from build123d import *

# Parameters (mm, degrees)
ESQUISSE2_R             = 3
ENL_V_MAT_EXTRU_2_DEPTH = 53.428729839


with BuildPart() as part:
    # Esquisse1 → Révolution1 (revolve)
    with BuildSketch(Plane.XY, mode=Mode.PRIVATE) as r_volution1_sk:
        Polygon((-4, 31.5125), (-5.08, 31.5125), (-5.08, 36.5125), (5.08, 36.5125), (5.08, 31.5125), (4, 31.5125), (4, 0), (-4, 0), align=None)
    revolve(r_volution1_sk.sketch.rotate(Axis((-4, 0, 0), (1, 0, 0)), 90), axis=Axis((-4, 0, 0), (1, 0, 0)))

    # Esquisse2 → Enlèv. mat.-Extru.2 (cut, through all)
    with BuildSketch(Plane(origin=(4, 0, 0), x_dir=(0, 0, -1), z_dir=(1, 0, 0))):
        Circle(ESQUISSE2_R)
    extrude(amount=-ENL_V_MAT_EXTRU_2_DEPTH, mode=Mode.SUBTRACT)


solid = part.part
Design review of the part built by this model. Coordinates are the model's own, in mm. A direction names the side the tool comes from. Give positions to 0.01 mm unless a question says otherwise; leave off trailing zeros. Order: outer loops, then holes, each group sorted by start corner. A loop starts at its lowest first (then second) coordinate and runs counter-clockwise, first axis right, second up.
1. Add section A-A, the plane z = 0. State the section outline as (x, y) points, then the cut area to 3 significant figures.
Solution:
outline: (-5.08, -36.51) - (5.08, -36.51) - (5.08, -31.51) - (4, -31.51) - (4, -3) - (-4, -3) - (-4, -31.51) - (-5.08, -31.51) - close; (-5.08, 31.51) - (-4, 31.51) - (-4, 3) - (4, 3) - (4, 31.51) - (5.08, 31.51) - (5.08, 36.51) - (-5.08, 36.51) - close
area: 558 mm2
2. Mouldability with a two-part tool opening along Z and no side actions: class faces 1 (the flat face through (5.08, 11, -30)), 2 (the cylindrical face through (-4.55, -1.39, -31.48)), 3 (the cylindrical face through (0.07, 32.39, 16.85)) as +Z half, -Z half, draft (parallel to the pull), parting line (faces both ways), or undercut.
Solution:
face 1: draft
face 2: undercut
face 3: parting line
3. For pin 1 Ø1 at (x, y) = (-2.5, 4.5) entering from +Z; pin 2 Ø2 at (x, y) = (-0.5, 24.5) entering from +Z; pin 3 Ø8 at (y, z) = (-12.5, 13.5) entering from +X, all flat-tipped, find the tip position at first contact; note any pin that passes through.
Solution:
pin 1: stops at z = 36.29
pin 2: stops at z = 27.94
pin 3: stops at x = 4
4. To check wall thickness, follow L1, parallel to Y at x = 4.8, z = 0; L2, parallel to X at y = 2.5, z = 15.5; L3, parallel to Z at x = -1.5, y = 0.5. State the ranges of each line that lie inside material, in increasing order.
Solution:
L1: y = -36.51 to -31.51, 31.51 to 36.51
L2: x = -4 to 4
L3: z = -36.51 to -2.96, 2.96 to 36.51
5. Add section D-D, the plane y = -27. State the section outline as (x, z) points, then the cut area to 3 significant figures.
Solution:
outline: (-5.08, -24.58) - (5.08, -24.58) - (5.08, -16.25) - (4, -16.25) - (4, 16.25) - (5.08, 16.25) - (5.08, 24.58) - (-5.08, 24.58) - (-5.08, 16.25) - (-4, 16.25) - (-4, -16.25) - (-5.08, -16.25) - close
area: 429 mm2
6. Add section C-C, the plane x = 1. State the section outline as (y, z) points (1 decimal), then the cut area to 3 significant figures.
Solution:
outline: circle Ø73 at (0, 0); hole circle Ø6 at (0, 0)
area: 4,160 mm2
7. Tool access review of faces 4 (the flat face through (-4, 7, 0)), 5 (the cylindrical face through (4.53, -1.39, -31.48)), 6 (the flat face through (-5.08, 11, 30)): name each direction out of +Z, -Z, +X, -X, +Y, -Y from which nothing blocks a thin tool from reaching the whole face with its end or side.
Solution:
face 4: -X
face 5: +X
face 6: +Z, -Z, -X, +Y, -Y
